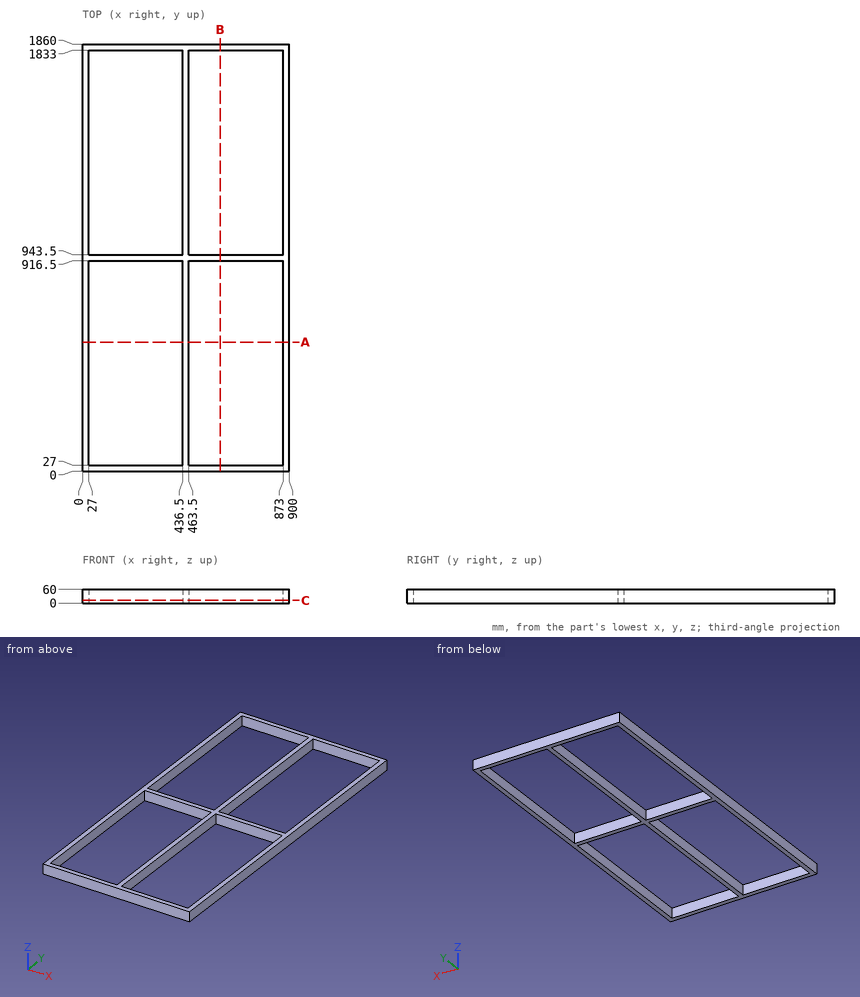
The drawing under review shows one solid part. Ordinate dimensions are in mm from its lowest x, y, z. Coordinates: 2 decimals unless noted, no trailing zeros. Write each loop counter-clockwise with the first axis right and the second up, starting at its lowest first coordinate (ties: lowest second). Pieces come first, ordered by that corner, then holes. Notation, with made-up numbers: M -32,65 L 27,65 A16 ccw 27,90 Z; hole C 12,-26.5 d6. An arc over 180 degrees is marked long. Answer as a JSON object with one key per item and string values.
Item 1: Add section A-A, the plane y = 562.5. Give the boundary of the cut face in (x, z).
Outcome:
{"outline": "M 0,0 L 27,0 L 27,60 L 0,60 Z; M 436.5,0 L 463.5,0 L 463.5,60 L 436.5,60 Z; M 873,0 L 900,0 L 900,60 L 873,60 Z"}
Item 2: Add section B-B, the plane x = 599.5. Give the boundary of the cut face in (y, z), and give its area (3 significant figures).
Outcome:
{"outline": "M 0,0 L 27,0 L 27,60 L 0,60 Z; M 916.5,0 L 943.5,0 L 943.5,60 L 916.5,60 Z; M 1833,0 L 1860,0 L 1860,60 L 1833,60 Z", "area": "4,860 mm²"}
Item 3: Add section C-C, the plane z = 12. Give the boundary of the cut face in (x, y).
Outcome:
{"outline": "M 0,0 L 900,0 L 900,1860 L 0,1860 Z; hole M 27,27 L 436.5,27 L 436.5,916.5 L 27,916.5 Z; hole M 27,943.5 L 436.5,943.5 L 436.5,1833 L 27,1833 Z; hole M 463.5,27 L 873,27 L 873,916.5 L 463.5,916.5 Z; hole M 463.5,943.5 L 873,943.5 L 873,1833 L 463.5,1833 Z"}
Item 4: Insertion check: pin 1 Ø1 at (x, z) = (371, 40.5) entering from -Y. The pin has a flat end and moves straight along its axis. Give the tip position at first contact, or say it passes through.
Outcome:
{"pin 1": "y = 0"}
Item 5: Wall thickness on probe 1 along Y at (x, z) = (654.5, 33.5); probe 2 along X at (y, z) = (414.5, 31): over which ranges is each line inside the solid? List them lowest first.
Outcome:
{"probe 1": "0 to 27, 916.5 to 943.5, 1833 to 1860", "probe 2": "0 to 27, 436.5 to 463.5, 873 to 900"}
